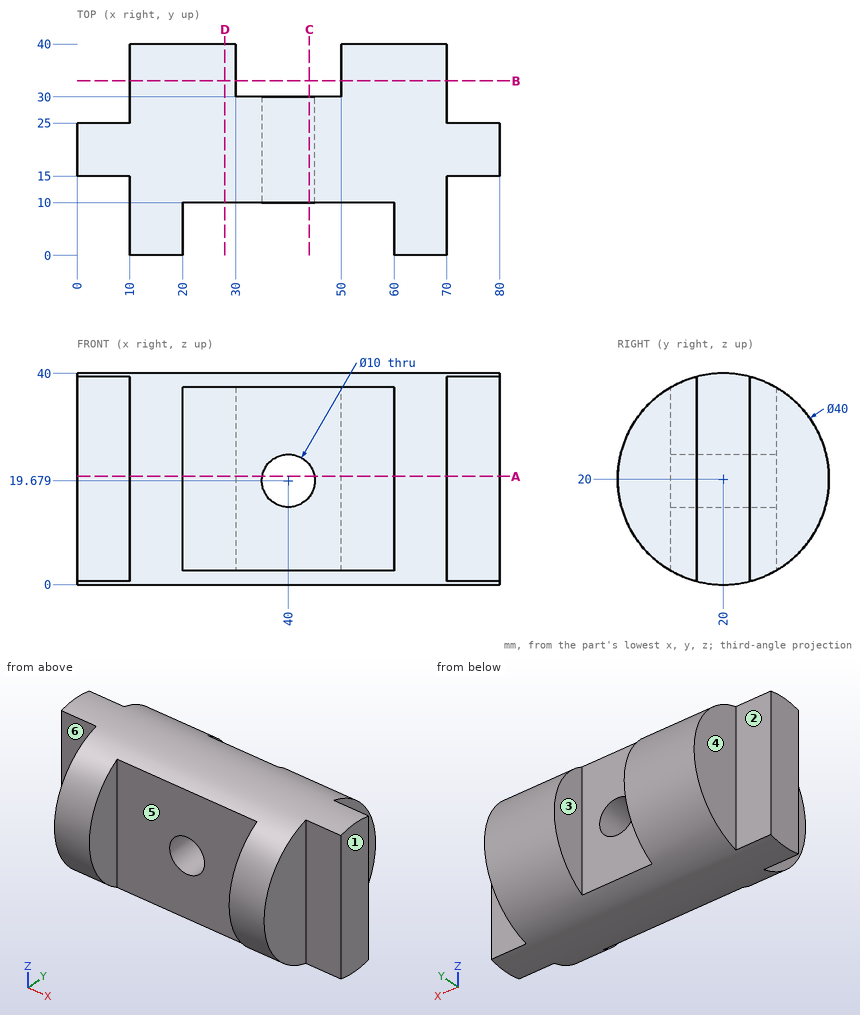
Study the drawing (mm; zero at the part's minimum x, y, z) and answer. A direction names the side the tool comes from. Coordinates: 2 decimals unless noted, no trailing zeros. Write each loop counter-clockwise with the first axis right and the second up, starting at its lowest first coordinate (ties: lowest second). Pieces come first, ordered by that corner, then holes. Notation, with made-up numbers: (39, 51) - (62, 51) arc R20 ccw to (62, 87) - close; hole circle Ø7 at (-31.5, -17.5). An arc over 180 degrees is marked (long way). Answer as a JSON object with one key per item and string values. Group by question number.
1. Each of these flat-tipped pins is pushed along its axis until it touches: P1, Ø6, axis at x = 40, z = 19.68, coming from the +Y side; P2, Ø11, axis at y = 37, z = 21.5, coming from the +X side; P3, Ø2, axis at x = 58.5, y = 23, coming from the +Z side; P4, Ø7.5, axis at y = 33.5, z = 22.5, coming from the -X side. Where does it stop, or does it pass through?
2. A cutting plane is placed at C-C (x = 44). Determine the outline of the cut face in (y, z).
3. Which of the six approach directions +Z, -Z, +X, -X, +Y, -Y give full straight-line access (tool end or side, diameter ignored) to the marked faces 4, 5 and 6?
4. A cutting plane is placed at B-B (y = 33). Determine the outline of the cut face in (x, z).
5. The mould has two halves that part along X. Classify the marked faces 1, 2 and 3: +X half, -X half, draft (parallel to the pull), parting line (faces both ways), or undercut.
6. A cutting plane is placed at D-D (x = 28). Determine the outline of the cut face in (y, z), plus the area to 3 significant figures.
7. Consider L1, parallel to X at y = 33, z = 25.5; L2, parallel to Z at x = 40, y = 15 (1 decimal); L3, parallel to Z at x = 57, y = 30. Determine where each line is inside the solid, lowest interval first. Write a range as [from, to].
8. A cutting plane is placed at A-A (z = 20.5). Determine the outline of the cut face in (x, y).
Worked out:
{
 "1": {"P1": "passes through", "P2": "stops at x = 70", "P3": "stops at z = 39.9", "P4": "stops at x = 10"},
 "2": {"outline": "(10, 2.68) arc R20 ccw to (30, 2.68) - (30, 16.68) - (10, 16.68) - close; (10, 22.68) - (30, 22.68) - (30, 37.32) arc R20 ccw to (10, 37.32) - close"},
 "3": {"face 4": "+Z, -Z, -X, +Y", "face 5": "+Z, -Z, -Y", "face 6": "+Z, -Z, -X, -Y"},
 "4": {"outline": "(10, 4.8) - (30, 4.8) - (30, 35.2) - (10, 35.2) - close; (50, 4.8) - (70, 4.8) - (70, 35.2) - (50, 35.2) - close"},
 "5": {"face 1": "+X half", "face 2": "draft", "face 3": "undercut"},
 "6": {"outline": "(10, 2.68) arc R20 ccw (long way) to (10, 37.32) - close", "area": "1,010 mm²"},
 "7": {"L1": "x = [10, 30], [50, 70]", "L2": "z = [0.6, 14.7], [24.7, 39.4]", "L3": "z = [2.68, 37.32]"},
 "8": {"outline": "(0, 15) - (10, 15) - (10, 0.01) - (20, 0.01) - (20, 10) - (35.07, 10) - (35.07, 30) - (30, 30) - (30, 39.99) - (10, 39.99) - (10, 25) - (0, 25) - close; (44.93, 10) - (60, 10) - (60, 0.01) - (70, 0.01) - (70, 15) - (80, 15) - (80, 25) - (70, 25) - (70, 39.99) - (50, 39.99) - (50, 30) - (44.93, 30) - close"}
}
